```python
from build123d import *

# Parameters (mm, degrees)
BOSS_EXTRUDE1_DEPTH = 530
CUT_EXTRUDE1_DEPTH  = 520
BOSS_EXTRUDE2_START = 10
BOSS_EXTRUDE2_DEPTH = 10
SKETCH4_W           = 120
SKETCH4_H           = 520
CUT_EXTRUDE2_DEPTH  = 313


with BuildPart() as part:
    # Sketch2 → Boss-Extrude1 (new body)
    with BuildSketch(Plane.XY):
        with BuildLine():
            Line((650, 0), (650, 224.276251584))
            ThreePointArc((650, 224.276251584), (643.051126749, 239.431055792), (627.033190941, 244.054978641))
            Line((627.033190941, 244.054978641), (17.033190941, 152.554978641))
            ThreePointArc((17.033190941, 152.554978641), (4.845195792, 145.827378333), (0, 132.776251584))
            Line((0, 132.776251584), (0, 0))
            Line((0, 0), (0, -10))
            Line((0, -10), (650, -10))
            Line((650, -10), (650, 0))
        make_face()
        with BuildLine():
            Line((660, -10), (660, 224.276251584))
            ThreePointArc((660, 224.276251584), (649.576690123, 247.008457896), (625.549786412, 253.94434217))
            Line((625.549786412, 253.94434217), (15.549786412, 162.44434217))
            ThreePointArc((15.549786412, 162.44434217), (-2.732206312, 152.352941707), (-10, 132.776251584))
            Line((-10, 132.776251584), (-10, -10))
            Line((-10, -10), (0, -10))
            Line((0, -10), (0, 0))
            Line((0, 0), (0, 132.776251584))
            ThreePointArc((0, 132.776251584), (4.845195792, 145.827378333), (17.033190941, 152.554978641))
            Line((17.033190941, 152.554978641), (627.033190941, 244.054978641))
            ThreePointArc((627.033190941, 244.054978641), (643.051126749, 239.431055792), (650, 224.276251584))
            Line((650, 224.276251584), (650, 0))
            Line((650, 0), (650, -10))
            Line((650, -10), (660, -10))
        make_face()
    extrude(amount=-BOSS_EXTRUDE1_DEPTH)

    # Sketch2_3 → Cut-Extrude1 (cut)
    with BuildSketch(Plane.XY):
        with BuildLine():
            Line((650, 0), (650, 224.276251584))
            ThreePointArc((650, 224.276251584), (643.051126749, 239.431055792), (627.033190941, 244.054978641))
            Line((627.033190941, 244.054978641), (17.033190941, 152.554978641))
            ThreePointArc((17.033190941, 152.554978641), (4.845195792, 145.827378333), (0, 132.776251584))
            Line((0, 132.776251584), (0, 0))
            Line((0, 0), (0, -10))
            Line((0, -10), (650, -10))
            Line((650, -10), (650, 0))
        make_face()
    extrude(amount=-CUT_EXTRUDE1_DEPTH, mode=Mode.SUBTRACT)

    # Sketch2_4 → Boss-Extrude2 (add)
    with BuildSketch(Plane.XY.offset(BOSS_EXTRUDE2_START)):
        with BuildLine():
            Line((660, -10), (660, 224.276251584))
            ThreePointArc((660, 224.276251584), (649.576690123, 247.008457896), (625.549786412, 253.94434217))
            Line((625.549786412, 253.94434217), (15.549786412, 162.44434217))
            ThreePointArc((15.549786412, 162.44434217), (-2.732206312, 152.352941707), (-10, 132.776251584))
            Line((-10, 132.776251584), (-10, -10))
            Line((-10, -10), (0, -10))
            Line((0, -10), (0, 0))
            Line((0, 0), (0, 132.776251584))
            ThreePointArc((0, 132.776251584), (4.845195792, 145.827378333), (17.033190941, 152.554978641))
            Line((17.033190941, 152.554978641), (627.033190941, 244.054978641))
            ThreePointArc((627.033190941, 244.054978641), (643.051126749, 239.431055792), (650, 224.276251584))
            Line((650, 224.276251584), (650, 0))
            Line((650, 0), (650, -10))
            Line((650, -10), (660, -10))
        make_face()
        with BuildLine():
            Line((650, 0), (650, 224.276251584))
            ThreePointArc((650, 224.276251584), (643.051126749, 239.431055792), (627.033190941, 244.054978641))
            Line((627.033190941, 244.054978641), (17.033190941, 152.554978641))
            ThreePointArc((17.033190941, 152.554978641), (4.845195792, 145.827378333), (0, 132.776251584))
            Line((0, 132.776251584), (0, 0))
            Line((0, 0), (0, -10))
            Line((0, -10), (650, -10))
            Line((650, -10), (650, 0))
        make_face()
    extrude(amount=-BOSS_EXTRUDE2_DEPTH)

    # Sketch4 → Cut-Extrude2 (cut)
    with BuildSketch(Plane(origin=(0, 0, 0), x_dir=(1, 0, 0), z_dir=(0, 1, 0))):
        with Locations((360, 260)):
            Rectangle(SKETCH4_W, SKETCH4_H)
    extrude(amount=CUT_EXTRUDE2_DEPTH, mode=Mode.SUBTRACT)


solid = part.part
```
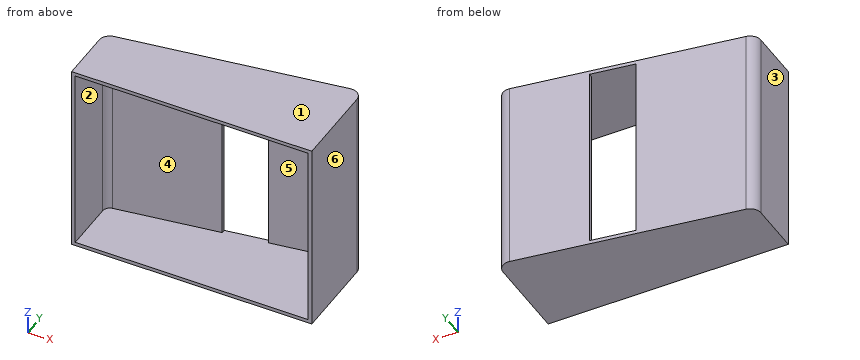
Input: part model. Units: mm. Frame: model coordinates. Face numbers are marked on the shaded views. A direction names the side the tool comes from. Round coordinates to 2 decimals unless told otherwise and drop trailing zeros. Loops run counter-clockwise (first coordinate to the right, second up) from the corner with the lowest first, then second, coordinate; pieces in that order, holes last. Notation, with made-up numbers: (-38.75, 61.5) - (-28.75, 61.5) arc R19 ccw to (-28.75, 85.5) - close; hole circle Ø2 at (80, -26). An arc over 180 degrees is marked (long way). One line per item, written item: value. Start each with the question number.
(1) Contact query for flat-ended pins moving along their axis: P1, Ø5, axis at x = 441.5, z = -66, coming from the -Y side; P2, Ø1, axis at x = 293, z = -62, coming from the -Y side (3 decimals); P3, Ø10, axis at x = 83, z = -243.5, coming from the -Y side. Output: stop coordinate, or through.
(2) Section B-B, the plane z = -117. Return loops of the section in (x, y), plus the area to 3 significant figures.
(3) Section D-D, the plane x = 566. Return loops of the section in (y, z), plus the area to 3 significant figures.
(4) Section A-A, the plane x = 378.5. Return loops of the section in (y, z), plus the area to 3 significant figures.
(5) Draft query along Z for the marked faces 1, 2, 3 and 4. Return one class per face: +Z half, -Z half, draft (parallel to the pull), parting line (faces both ways), or undercut.
(6) Section C-C, the plane y = 105. Return loops of the section in (x, z), plus the area to 3 significant figures.
(7) Access query for the marked faces 5 and 6. Directions: +Z, -Z, +X, -X, +Y, -Y. A direction counts if a zero-diameter tool reaches every point of the face in a straight line with its end or side. Return the directions, or none.
(8) Ray query, line 1 (X direction, y = 30, z = -206.5); line 2 (Z direction, x = 274.5, y = 120); line 3 (X direction, y = 135, z = -277). Return the intervals inside material, ascending. Write a range as [from, to].
Results below:
1. P1: y = 215.85
1. P2: y = 193.875
1. P3: y = 161.7
2. outline: (-10, -10) - (0, -10) - (0, 132.78) arc R20 cw to (17.03, 152.55) - (300, 195) - (300, 205.11) - (15.55, 162.44) arc R30 ccw to (-10, 132.78) - close; (420, 213) - (627.03, 244.05) arc R20 cw to (650, 224.28) - (650, -10) - (660, -10) - (660, 224.28) arc R30 ccw to (625.55, 253.94) - (420, 223.11) - close
2. area: 9,510 mm^2
3. outline: (-10, -530) - (245.01, -530) - (245.01, 10) - (-10, 10) - (-10, 0) - (234.9, 0) - (234.9, -520) - (-10, -520) - close
3. area: 10,400 mm^2
4. outline: (-10, -530) - (216.89, -530) - (216.89, -520) - (-10, -520) - close; (-10, 0) - (216.89, 0) - (216.89, 10) - (-10, 10) - close
4. area: 4,540 mm^2
5. face 1: +Z half
5. face 2: undercut
5. face 3: draft
5. face 4: undercut
6. outline: (-10, -530) - (660, -530) - (660, 10) - (-10, 10) - close; hole (0, -520) - (650, -520) - (650, 0) - (0, 0) - close
6. area: 23,800 mm^2
7. face 5: -Y
7. face 6: +Z, -Z, +X, +Y, -Y
8. line 1: [-10, 0], [650, 660]
8. line 2: [-530, -520], [0, 10]
8. line 3: [-9.92, 0.12], [650, 660]
